The listing builds one solid part. Answer for the finished solid, in the listing's coordinates (mm). Face numbers are marked on the shaded views. Coordinates: 2 decimals unless noted, no trailing zeros. Loops run counter-clockwise (first coordinate to the right, second up) from the corner with the lowest first, then second, coordinate; pieces in that order, holes last. Notation, with made-up numbers: M -24,55.5 L 31,55.5 A27 ccw 31,72.5 Z; hole C 63,82 d8. An arc over 180 degrees is marked long. Return JSON: item names as keys, results as strings. Group by question number.
1. The mould has two halves that part along Z. Classify the marked faces 1, 2 and 3: pulls with the +Z half, pulls with the -Z half, needs draft (parallel to the pull), parting line crosses it, or undercut.
2. Straight lines are drawn through the part: L1, parallel to X at y = -47.5, z = 36 (1 decimal); L2, parallel to Z at x = 2, y = -19; L3, parallel to Z at x = 10, y = -41.5. For each, find the intervals that lie inside material, in ascending order. Write a range as from..to.
3. Section D-D (x = 14) is taken. Write down the section's boundary in (y, z), then the cut area to 3 significant figures.
4. Given P1, Ø10, axis at x = 41.5, y = 32, coming from the +Z side; P2, Ø5, axis at x = -19, y = -18.5, coming from the -Z side; P3, Ø12, axis at y = 12, z = 25.5, coming from the +X side (3 decimals); P4, Ø9, axis at x = 49.5, z = 28.5, coming from the +Y side, each flat-ended and moving along its own axis, determine where each tip first touches the part or whether it passes through.
5. Section A-A (x = -35) is taken. Write down the section's boundary in (y, z).
6. Section B-B (y = 27.5) is taken. Write down the section's boundary in (x, z) (1 decimal).
7. Section C-C (z = 32) is taken. Count the separate pieces of the cut face and the enclosed holes in it, then the cut area to 3 significant figures.
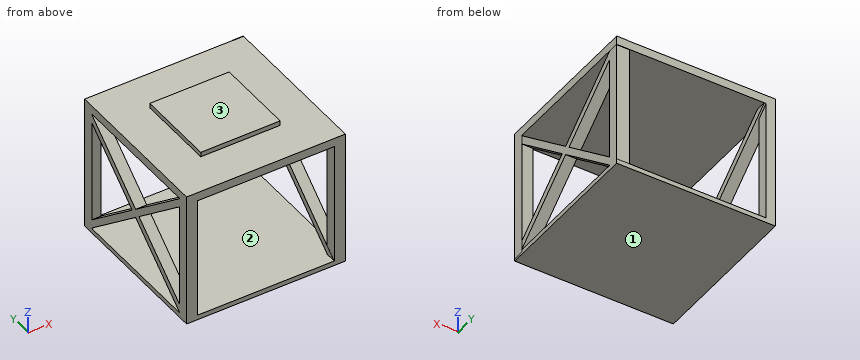
```python
from build123d import *

# Parameters (mm, degrees)
F0_W      = 100
F0_H      = 100
F1_DEPTH  = 3
F3_DEPTH  = 7
F5_DEPTH  = 7
F7_DEPTH  = 7
F9_DEPTH  = 7
F10_W     = 100.0225
F10_H     = 5.475754
F11_DEPTH = 100
F12_W     = 50.0005
F12_H     = 50
F13_DEPTH = 3
F14_W     = 5.79754
F14_H     = 7
F14_W_2   = 8.194392
F14_W_3   = 7
F15_DEPTH = 84.1


with BuildPart() as f1:
    # F0 (on Top) → F1 (new body)
    with BuildSketch(Plane.XY):
        with Locations((5.625, -3.024291)):
            Rectangle(F0_W, F0_H)
    extrude(amount=F1_DEPTH)

    # F2 (on face) → F3 (join)
    with BuildSketch(Plane(origin=(-44.375, 0, 0), x_dir=(0, -1, 0), z_dir=(-1, 0, 0))):
        Polygon((-46.975709, 0), (-43.975709, 0), (53.024291, 80.049396), (53.024291, 85.52515), (-46.975709, 3), align=None)
    extrude(amount=-F3_DEPTH)

    # F4 (on face) → F5 (join)
    with BuildSketch(Plane(origin=(-44.375, 0, 0), x_dir=(0, -1, 0), z_dir=(-1, 0, 0))):
        Polygon((-46.975709, 80.049396), (50.024291, 0), (53.024291, 0), (53.024291, 3), (-46.975709, 85.52515), align=None)
    extrude(amount=-F5_DEPTH)

    # F6 (on face) → F7 (join)
    with BuildSketch(Plane.YZ.offset(55.625)):
        Polygon((-53.024291, 0), (-50.024291, 0), (46.975709, 80.049396), (46.975709, 85.644148), (-53.024291, 3), align=None)
    extrude(amount=-F7_DEPTH)

    # F8 (on face) → F9 (join)
    with BuildSketch(Plane.YZ.offset(55.625)):
        Polygon((-53.024291, 80.049396), (43.975709, 0), (46.975709, 0), (46.975709, 3), (-53.024291, 85.554466), align=None)
    extrude(amount=-F9_DEPTH)

    # F10 (on face) → F11 (join)
    with BuildSketch(Plane.XZ.offset(53.024291)):
        with Locations((5.63625, 82.787273)):
            Rectangle(F10_W, F10_H)
    extrude(amount=-F11_DEPTH)

    # F12 (on face) → F13 (join)
    with BuildSketch(Plane.XY.offset(85.52515)):
        with Locations((5.62525, -3.024291)):
            Rectangle(F12_W, F12_H)
    extrude(amount=F13_DEPTH)

    # F14 (on face) → F15 (join)
    with BuildSketch(Plane.XY.offset(85.52515)):
        with Locations((-41.47623, 43.475709)):
            Rectangle(F14_W, F14_H)
        with Locations((51.527804, 43.33172)):
            Rectangle(F14_W_2, F14_H)
        with Locations((52.1475, -49.524291)):
            Rectangle(F14_W_3, F14_H)
        with Locations((-40.875, -49.524291)):
            Rectangle(F14_W_3, F14_H)
    extrude(amount=-F15_DEPTH)


solid = f1.part
```
Worked out:
{
 "1": {"face 1": "pulls with the -Z half", "face 2": "undercut", "face 3": "pulls with the +Z half"},
 "2": {"L1": "-44.4..-37.4, 48.6..55.6", "L2": "0..3, 80.05..88.53", "L3": "0..3, 80.05..85.53"},
 "3": {"outline": "M -53.02,0 L 46.98,0 L 46.98,3 L -53.02,3 Z; M -53.02,80.05 L 46.98,80.05 L 46.98,85.53 L 21.98,85.53 L 21.98,88.53 L -28.02,88.53 L -28.02,85.53 L -53.02,85.53 Z", "area": "998 mm^2"},
 "4": {"P1": "z = 85.53", "P2": "z = 0", "P3": "x = 55.625", "P4": "y = 46.83"},
 "5": {"outline": "M -53.02,0 L 46.98,0 L 46.98,3 L -53.02,3 Z; M -53.02,80.05 L 46.98,80.05 L 46.98,85.53 L -53.02,85.53 Z"},
 "6": {"outline": "M -44.4,0 L 55.6,0 L 55.6,3 L -44.4,3 Z; M -44.4,13.6 L -37.4,13.6 L -37.4,19.1 L -44.4,19.1 Z; M -44.4,64 L -37.4,64 L -37.4,69.5 L -44.4,69.5 Z; M -44.4,80 L 55.6,80 L 55.6,85.5 L -44.4,85.5 Z; M 48.6,13.6 L 55.6,13.6 L 55.6,19.1 L 48.6,19.1 Z; M 48.6,64 L 55.6,64 L 55.6,69.5 L 48.6,69.5 Z"},
 "7": {"separate pieces": "8", "enclosed holes": "0", "area": "382 mm^2"}
}
